Read the model definition and answer for the solid it produces. Units are mm, in the model's axes. Face numbers are marked on the shaded views. A direction names the side the tool comes from. Coordinates: 2 decimals unless noted, no trailing zeros. Loops run counter-clockwise (first coordinate to the right, second up) from the corner with the lowest first, then second, coordinate; pieces in that order, holes last. Notation, with made-up numbers: (29, 69.5) - (59, 69.5) arc R36 cw to (59, 106.5) - close; hole circle Ø8 at (61.25, -26). An arc over 180 degrees is marked (long way). Use one line per item in the form item = value.
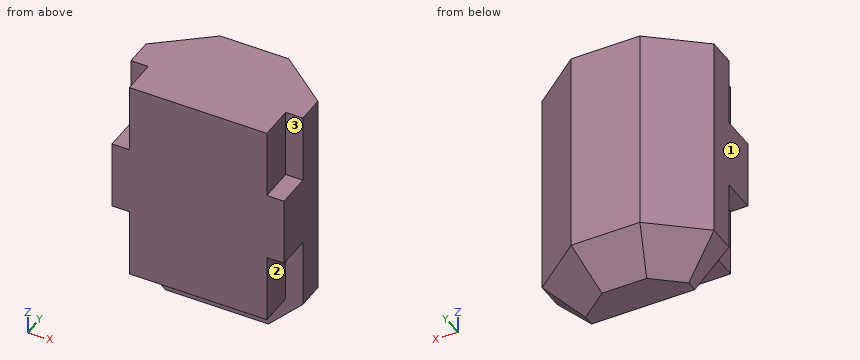
from build123d import *

# Parameters (mm, degrees)
BOSS_EXTRU_1_DEPTH = 600
ESQUISSE2_W        = 200
ESQUISSE2_H        = 100
BOSS_EXTRU_2_DEPTH = 500
BOSS_EXTRU_3_DEPTH = 100
CHANFREIN1_SIZE    = 100


with BuildPart() as part:
    # Esquisse1 → Boss.-Extru.1 (new body)
    with BuildSketch(Plane.XY):
        Polygon((-250, 30), (-100, 150), (100, 150), (250, 30), (250, -50), (200, -50), (200, -150), (-200, -150), (-200, -50), (-250, -50), align=None)
    extrude(amount=BOSS_EXTRU_1_DEPTH)

    # Esquisse2 → Boss.-Extru.2 (add)
    with BuildSketch(Plane.ZY.offset(250)):
        with Locations((300, -100)):
            Rectangle(ESQUISSE2_W, ESQUISSE2_H)
    extrude(amount=-BOSS_EXTRU_2_DEPTH)

    # Esquisse3 → Boss.-Extru.3 (add)
    with BuildSketch(Plane(origin=(0, 0, 0), x_dir=(-1, 0, 0), z_dir=(0, 0, -1))):
        Polygon((-200, -50), (200, -50), (250, -50), (250, 30), (100, 150), (-100, 150), (-250, 30), (-250, -50), align=None)
    extrude(amount=BOSS_EXTRU_3_DEPTH)

    # Chanfrein1
    chanfrein1_edges = [part.edges().sort_by_distance(p)[0] for p in [
        (-250, -10, -100),
        (-175, 90, -100),
        (0, 150, -100),
        (175, 90, -100),
        (250, -10, -100),
    ]]
    chamfer(chanfrein1_edges, length=CHANFREIN1_SIZE)


solid = part.part
Item 1: Find the intervals of material crossed by L1, parallel to Z at x = -219.5, y = -57; L2, parallel to X at y = -59, z = 427; L3, parallel to Z at x = -198.5, y = -57, in increasing order.
Results below:
L1 = 200 to 400
L2 = -200 to 200
L3 = 0 to 600
Item 2: The part is cut by section D-D on x = -112. Give the vertices of the cut face in (y, z).
Results below:
outline = (-150, 0) - (-50, 0) - (-50, -100) - (12.34, -100) - (140.4, 0) - (140.4, 600) - (-150, 600) - close
Item 3: The part is cut by section A-A on y = -122. Give the vertices of the cut face in (x, z), plus the area to 3 significant figures.
Results below:
outline = (-250, 200) - (-200, 200) - (-200, 0) - (200, 0) - (200, 200) - (250, 200) - (250, 400) - (200, 400) - (200, 600) - (-200, 600) - (-200, 400) - (-250, 400) - close
area = 260,000 mm²
Item 4: The part is cut by section C-C on x = -3. Give the vertices of the cut face in (y, z).
Results below:
outline = (-150, 0) - (-50, 0) - (-50, -100) - (50, -100) - (150, 0) - (150, 600) - (-150, 600) - close
Item 5: Each of these flat-tipped pins is pushed along its axis until it touches: P1, Ø15, axis at x = -236, z = 531.5, coming from the -Y side; P2, Ø25, axis at x = 226, y = -116, coming from the -Z side; P3, Ø1, axis at x = 197.5, y = -119, coming from the -Z side. Where does it stop, or does it pass through?
Results below:
P1 = -50
P2 = 200
P3 = 0
Item 6: Which of the six approach directions +Z, -Z, +X, -X, +Y, -Y give full straight-line access (tool end or side, diameter ignored) to the marked faces 1, 2 and 3?
Results below:
face_1 = +Z, -Z, -X, +Y, -Y
face_2 = -Z, +X, -Y
face_3 = +Z, +X, -Y
Item 7: The part is cut by section B-B on z = 132. Give the vertices of the cut face in (x, y).
Results below:
outline = (-250, -50) - (-200, -50) - (-200, -150) - (200, -150) - (200, -50) - (250, -50) - (250, 30) - (100, 150) - (-100, 150) - (-250, 30) - close
